Read the model definition and answer for the solid it produces. Units are mm, in the model's axes. A direction names the side the tool comes from. Coordinates: 2 decimals unless noted, no trailing zeros. Write each loop counter-clockwise with the first axis right and the second up, starting at its lowest first coordinate (ties: lowest second). Pieces come first, ordered by that corner, then holes. Notation, with made-up numbers: (9, 29.5) - (61, 29.5) arc R16 ccw to (61, 34.5) - close; hole circle Ø5 at (10.5, 10). An arc over 180 degrees is marked (long way). Return JSON: item names as keys, results as strings.
```python
from build123d import *

# Parameters (mm, degrees)
F0_R        = 38.1
F0_R_2      = 23.8125
F1_DEPTH    = 12.7
F0_R_3      = 44.45
F1_FACE_R   = 38.1
F1_FACE_R_2 = 23.8125
F2_DEPTH    = 6.35
F3_SIZE     = 3.175
F4_SIZE     = 0.8128


with BuildPart() as f1:
    # F0 (on Top) → F1 (new body)
    with BuildSketch(Plane.XY):
        Circle(F0_R)
        Circle(F0_R_2, mode=Mode.SUBTRACT)
    extrude(amount=-F1_DEPTH)

    # F0 (on Top) + F1_face (on face) → F2 (join)
    with BuildSketch(Plane.XY):
        Circle(F0_R_3)
        Circle(F0_R, mode=Mode.SUBTRACT)
    with BuildSketch(Plane.XY):
        Circle(F1_FACE_R)
        Circle(F1_FACE_R_2, mode=Mode.SUBTRACT)
    extrude(amount=F2_DEPTH)

    # F3
    f3_edges = [f1.edges().sort_by_distance(p)[0] for p in [
        (-23.8125, 0, 6.35),
    ]]
    chamfer(f3_edges, length=F3_SIZE)

    # F4
    f4_edges = [f1.edges().sort_by_distance(p)[0] for p in [
        (-44.45, 0, 6.35),
        (-44.45, 0, 0),
        (-38.1, 0, -12.7),
    ]]
    chamfer(f4_edges, length=F4_SIZE)


solid = f1.part
```
(1) Flat-ended cylindrical pins translate along their axes: P1, Ø6, axis at y = 1.5, z = -9.5, coming from the +X side; P2, Ø5, axis at y = 33, z = 4.5, coming from the +X side (3 decimals); P3, Ø10, axis at x = -16, z = -0.5, coming from the -Y side. Find the tip coordinate at first contact, or state that the pin passes through.
Answer:
{"P1": "x = 38.1", "P2": "x = 32.335", "P3": "y = -43.02"}
(2) Straight lines are drawn through the part: line 1 (Y direction, x = 0, z = -8.75); line 2 (X direction, y = 9.5, z = 1.5); line 3 (Y direction, x = -2.5, z = 5.75). For each, find the intervals that lie inside material, in ascending order. Write a range as from..to.
Answer:
{"line 1": "-38.1..-23.81, 23.81..38.1", "line 2": "-43.42..-21.84, 21.84..43.42", "line 3": "-44.17..-26.27, 26.27..44.17"}
(3) Which of the six approach directions +Z, -Z, +X, -X, +Y, -Y give full straight-line access (tool end or side, diameter ignored) to faces 4 (the face through (22.86, 7.2, 3.33)), 5 (the face through (0, -39, 0))?
Answer:
{"face 4": "+Z", "face 5": "-Z"}
(4) Determine the mould class of faces 1 (the face through (-18.897, -14.49, -4.874)), 2 (the face through (-30.235, -23.183, -5.86)), 3 (the face through (-20, -19, 6.35)) for opening direction X: +X half, -X half, draft (parallel to the pull), parting line (faces both ways), or undercut.
Answer:
{"face 1": "undercut", "face 2": "parting line", "face 3": "draft"}
(5) A cutting plane is placed at C-C (z = -5). Determine the outline of the cut face in (x, y) (1 decimal), and give its area (3 significant figures).
Answer:
{"outline": "circle Ø76.2 at (0, 0); hole circle Ø47.6 at (0, 0)", "area": "2,780 mm²"}
